```python
from build123d import *

# Parameters (mm, degrees)
SKETCH1_W           = 89.156
SKETCH1_H           = 23
SKETCH1_R           = 10.25
BOSS_EXTRUDE1_DEPTH = 3.2
FILLET1_R           = 3


with BuildPart() as part:
    # Sketch1 → Boss-Extrude1 (new body)
    with BuildSketch(Plane(origin=(0, 0, 0), x_dir=(1, 0, 0), z_dir=(0, 1, 0))):
        Rectangle(SKETCH1_W, SKETCH1_H)
        with Locations(Location((30.328, 0, 0), (0, 0, 270))):
            Circle(SKETCH1_R, mode=Mode.SUBTRACT)
        with Locations(Location((-30.328, 0, 0), (0, 0, 270))):
            Circle(SKETCH1_R, mode=Mode.SUBTRACT)
    extrude(amount=BOSS_EXTRUDE1_DEPTH)

    # Fillet1
    fillet1_edges = [part.edges().sort_by_distance(p)[0] for p in [
        (44.578, 1.6, -11.5),
        (44.578, 1.6, 11.5),
        (-44.578, 1.6, 11.5),
        (-44.578, 1.6, -11.5),
    ]]
    fillet(fillet1_edges, radius=FILLET1_R)


solid = part.part
```
Build history of the part. All positions in model axes, mm. Round coordinates to 2 decimals unless told otherwise and drop trailing zeros. Write each loop counter-clockwise with the first axis right and the second up, starting at its lowest first coordinate (ties: lowest second). Pieces come first, ordered by that corner, then holes.
1) Band-saw the part on C-C, the plane y = 1.9. List the corners of the cut face in (x, z), and give its area (3 significant figures).
2) Band-saw the part on B-B, the plane x = -28. List the corners of the cut face in (y, z).
3) Band-saw the part on A-A, the plane z = 0. List the corners of the cut face in (x, y), and give its area (3 significant figures).
4) Drill centre lines: probe 1 along X at (y, z) = (1.75, 0); probe 2 along X at (y, z) = (1.15, 5); probe 3 along Z at (x, y) = (-38.5, 1.1). Where is each one in solid material? Low to high.
5) Mould opens along Z. For faces 1 (the flat face through (-1, 2, -11.5)), 2 (the flat face through (-1, 0, 0)), 3 (the cylindrical face through (-40.334, 1.578, -2.222)) say: +Z half, -Z half, draft (parallel to the pull), parting line (faces both ways), or undercut.
6) Band-saw the part on D-D, the plane z = -6.5. List the corners of the cut face in (x, y).
Ans:
1. outline: (-44.58, -8.5) arc R3 ccw to (-41.58, -11.5) - (41.58, -11.5) arc R3 ccw to (44.58, -8.5) - (44.58, 8.5) arc R3 ccw to (41.58, 11.5) - (-41.58, 11.5) arc R3 ccw to (-44.58, 8.5) - close; hole circle Ø20.5 at (-30.33, 0); hole circle Ø20.5 at (30.33, 0)
1. area: 1,380 mm2
2. outline: (0, -11.5) - (3.2, -11.5) - (3.2, -9.98) - (0, -9.98) - close; (0, 9.98) - (3.2, 9.98) - (3.2, 11.5) - (0, 11.5) - close
3. outline: (-44.58, 0) - (-40.58, 0) - (-40.58, 3.2) - (-44.58, 3.2) - close; (-20.08, 0) - (20.08, 0) - (20.08, 3.2) - (-20.08, 3.2) - close; (40.58, 0) - (44.58, 0) - (44.58, 3.2) - (40.58, 3.2) - close
3. area: 154 mm2
4. probe 1: x = -44.58 to -40.58, -20.08 to 20.08, 40.58 to 44.58
4. probe 2: x = -44.58 to -39.28, -21.38 to 21.38, 39.28 to 44.58
4. probe 3: z = -11.5 to -6.19, 6.19 to 11.5
5. face 1: -Z half
5. face 2: draft
5. face 3: undercut
6. outline: (-44.58, 0) - (-38.25, 0) - (-38.25, 3.2) - (-44.58, 3.2) - close; (-22.4, 0) - (22.4, 0) - (22.4, 3.2) - (-22.4, 3.2) - close; (38.25, 0) - (44.58, 0) - (44.58, 3.2) - (38.25, 3.2) - close
